```python
from build123d import *

# Parameters (mm, degrees)
BOSS_EXTRUDE1_DEPTH     = 22
CUT_EXTRUDE1_DEPTH      = 281.757902827
CUT_EXTRUDE1_DEPTH_BACK = 281.757902827
SKETCH3_R               = 2


with BuildPart() as part:
    # Sketch1 → Boss-Extrude1 (new, symmetric)
    with BuildSketch(Plane.XY):
        with BuildLine():
            Line((-50, 0), (50, 0))
            ThreePointArc((50, 0), (95.82575695, 30), (86.66060556, 84))
            ThreePointArc((86.66060556, 84), (68.99545417, 84.66515139), (68.33030278, 67))
            ThreePointArc((68.33030278, 67), (59.130783934, 26.727080442), (25, 50))
            Line((25, 50), (25, 151))
            Line((25, 151), (-25, 151))
            Line((-25, 151), (-25, 50))
            ThreePointArc((-25, 50), (-59.130783934, 26.727080442), (-68.33030278, 67))
            ThreePointArc((-68.33030278, 67), (-68.99545417, 84.66515139), (-86.66060556, 84))
            ThreePointArc((-86.66060556, 84), (-95.82575695, 30), (-50, 0))
        make_face()
    extrude(amount=BOSS_EXTRUDE1_DEPTH, both=True)

    # Sketch2 → Revolve1 (revolve)
    with BuildSketch(Plane.XY, mode=Mode.PRIVATE) as revolve1_sk:
        Polygon((0, 151), (35, 151), (35, 160), (20, 160), (20, 226), (15, 226), (15, 260), (0, 260), align=None)
    revolve(revolve1_sk.sketch.rotate(Axis((0, 260, 0), (0, -1, 0)), 180), axis=Axis((0, 260, 0), (0, -1, 0)))

    # Sketch3 → Cut-Extrude1 (cut, two sides: drawn at the far end of the back side and taken through both)
    with BuildSketch(Plane.XY.offset(-CUT_EXTRUDE1_DEPTH_BACK)):
        with Locations((0, 247.5)):
            Circle(SKETCH3_R)
    extrude(amount=CUT_EXTRUDE1_DEPTH + CUT_EXTRUDE1_DEPTH_BACK, mode=Mode.SUBTRACT)


solid = part.part
```
Geometry check sheet. Reference: the model listing, model coordinates, mm. A direction names the side the tool comes from. Coordinates: 2 decimals unless noted, no trailing zeros. Loops run counter-clockwise (first coordinate to the right, second up) from the corner with the lowest first, then second, coordinate; pieces in that order, holes last.
Item 1: Sectioned sample at D-D, the plane z = 29. Record the boundary of the cut face in (x, y), then the cut area to 3 significant figures.
Item 2: Sectioned sample at C-C, the plane y = 210.5. Record the boundary of the cut face in (x, z).
Item 3: Go/stop test with flat-tipped pins: pin 1 Ø3 at (x, z) = (-26, 18) entering from +Y; pin 2 Ø1.5 at (x, z) = (-76.5, 2) entering from +Y; pin 3 Ø8 at (y, z) = (170.5, 8.5) entering from -X. Record where each tip stops, or that it passes through.
Item 4: Thickness scan on line 1 (X direction, y = 50, z = -10.5); line 2 (X direction, y = 59.5, z = 10); line 3 (Y direction, x = 9, z = -20). Record the ranges inside material, lowest first.
Item 5: Sectioned sample at A-A, the plane y = 32.5. Record the boundary of the cut face in (x, z).
Item 6: Access from +Z, -Z, +X, -X, +Y, -Y to the whole of each face (thin tool, end or side, straight path). Record for faces 5 (the face through (-1, 60, -22)), 6 (the face through (25, 100, 0)), 7 (the face through (-3, 226, -15)), 8 (the face through (-1, 60, 22)).
Item 7: Sectioned sample at B-B, the plane y = 75. Record the boundary of the cut face in (x, z), then the cut area to 3 significant figures.
Item 8: Release check for a two-part mould opening along X. For faces 1 (the face through (69.2, 84.85, 0.31)), 2 (the face through (-1, 0, 0)), 3 (the face through (-25, 101, 0)), 4 (the face through (95.495, 29.259, 0.308)) record: released by +X, released by -X, zero draft, split by the parting line, or undercut.
Check result:
1. outline: (-19.6, 151) - (19.6, 151) - (19.6, 160) - (-19.6, 160) - close
1. area: 353 mm2
2. outline: circle Ø40 at (0, 0)
3. pin 1: stops at y = 160
3. pin 2: stops at y = 88
3. pin 3: stops at x = -19.49
4. line 1: x = -100 to -75, -25 to 25, 75 to 100
4. line 2: x = -99.09 to -73.12, -25 to 25, 73.12 to 99.09
4. line 3: y = 0 to 160
5. outline: (-96.84, -22) - (-67.85, -22) - (-67.85, 22) - (-96.84, 22) - close; (-32.15, -22) - (32.15, -22) - (32.15, 22) - (-32.15, 22) - close; (67.85, -22) - (96.84, -22) - (96.84, 22) - (67.85, 22) - close
6. face 5: -Z, +X, -X, -Y
6. face 6: +Z, -Z
6. face 7: +Y
6. face 8: +Z, +X, -X, -Y
7. outline: (-93.3, -22) - (-65.01, -22) - (-65.01, 22) - (-93.3, 22) - close; (-25, -22) - (25, -22) - (25, 22) - (-25, 22) - close; (65.01, -22) - (93.3, -22) - (93.3, 22) - (65.01, 22) - close
7. area: 4,690 mm2
8. face 1: undercut
8. face 2: zero draft
8. face 3: undercut
8. face 4: released by +X
